```python
from build123d import *

# Parameters (mm, degrees)
SKETCH_R  = 3
PAD_DEPTH = 10


with BuildPart() as part:
    # Sketch → Pad (new body)
    with BuildSketch(Plane.XY):
        with BuildLine():
            Line((128, 8), (0, 8))
            ThreePointArc((0, 8), (-7.799464, 1.77999), (-3.470741, -7.207909))
            Line((-3.470741, -7.207909), (29.963102, -23.306921))
            ThreePointArc((29.963102, -23.306921), (34.757227, -23.775851), (38.719233, -21.036134))
            ThreePointArc((85, -3), (59.145702, -5.054156), (38.719233, -21.036134))
            ThreePointArc((85, -3), (107.208893, -5.005497), (129.281329, -1.833032))
            ThreePointArc((129.281329, -1.833032), (132.958082, 3.646081), (128, 8))
        make_face()
        with Locations((33, -17)):
            Circle(SKETCH_R, mode=Mode.SUBTRACT)
        Circle(SKETCH_R, mode=Mode.SUBTRACT)
    extrude(amount=PAD_DEPTH)


solid = part.part
```
The listing builds one solid part. Answer for the finished solid, in the listing's coordinates (mm). Coordinates: 2 decimals unless noted, no trailing zeros. Loops run counter-clockwise (first coordinate to the right, second up) from the corner with the lowest first, then second, coordinate; pieces in that order, holes last. Notation, with made-up numbers: (33, -26) - (45, -26) arc R18 ccw to (45, -9) - close; hole circle Ø4 at (52, 13.25). An arc over 180 degrees is marked (long way). Use a Markdown table: item, result. Add a question column.
1) The part is cut by section A-A, the plane x = 33. Give the vertices of the cut face in (y, z).
2) The part is cut by section B-B, the plane y = 0. Give the vertices of the cut face in (x, z).
3) The part is cut by section D-D, the plane y = -12.5. Give the vertices of the cut face in (x, z), and give its area (3 significant figures).
4) Given pin 1 (1.5 mm diameter, centred on y = -12.5, z = 3.5, fed in from -X); pin 2 (5 mm diameter, centred on x = 33, y = -17, fed in from -Z); pin 3 (1.5 mm diameter, centred on x = 19.5, z = 5.5, fed in from -Y); pin 4 (3 mm diameter, centred on x = 70, z = 4.5, fed in from -Y), each flat-ended and moving along its own axis, determine where each tip first touches the part or whether it passes through.
5) Find the intervals of material crossed by line 1 (Y direction, x = 33, z = 5.5); line 2 (X direction, y = -19.5, z = 0.5); line 3 (X direction, y = -16, z = 0.5), in increasing order.
6) The mould has two halves that part along X. Classify faces 1 (the cylindrical face through (30.6, -18.8, 4.9)), 2 (the flat face through (13.012, -15.145, 4.93)), 3 (the cylindrical face through (-3, 0, 5)), 4 (the flat face through (65, 8, 5)): released by +X, released by -X, zero draft, split by the parting line, or undercut.
7) The part is cut by section C-C, the plane x = 51. Give the vertices of the cut face in (y, z), and give its area (3 significant figures).
Here are the results:
| question | item | result |
|---|---|---|
| 1 | outline | (-24, 0) - (-20, 0) - (-20, 10) - (-24, 10) - close; (-14, 0) - (8, 0) - (8, 10) - (-14, 10) - close |
| 2 | outline | (-8, 0) - (-3, 0) - (-3, 10) - (-8, 10) - close; (3, 0) - (132, 0) - (132, 10) - (3, 10) - close |
| 3 | outline | (7.52, 0) - (46.57, 0) - (46.57, 10) - (7.52, 10) - close |
| 3 | area | 391 mm^2 |
| 4 | pin 1 | stops at x = 5.96 |
| 4 | pin 2 | passes through |
| 4 | pin 3 | stops at y = -18.63 |
| 4 | pin 4 | stops at y = -2.53 |
| 5 | line 1 | y = -24 to -20, -14 to 8 |
| 5 | line 2 | x = 22.06 to 31.34, 34.66 to 39.85 |
| 5 | line 3 | x = 14.79 to 30.17, 35.83 to 42.85 |
| 6 | face 1 | undercut |
| 6 | face 2 | released by -X |
| 6 | face 3 | undercut |
| 6 | face 4 | zero draft |
| 7 | outline | (-9.23, 0) - (8, 0) - (8, 10) - (-9.23, 10) - close |
| 7 | area | 172 mm^2 |
